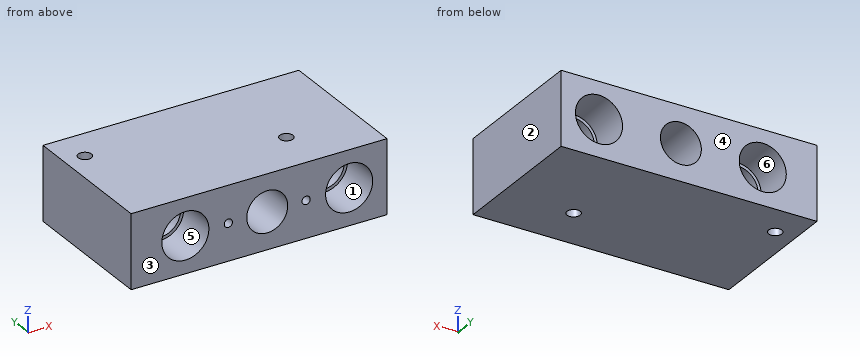
from build123d import *

# Parameters (mm, degrees)
F0_W      = 125
F0_H      = 70
F1_DEPTH  = 36
F2_R      = 10
F3_DEPTH  = 70.001
F4_R      = 11.5
F5_DEPTH  = 20
F6_R      = 11.5
F7_DEPTH  = 20
F8_R      = 3.25
F8_R_2    = 12.900097
F9_DEPTH  = 36.001
F10_R     = 2
F11_DEPTH = 20


with BuildPart() as f1:
    # F0 (on Top) → F1 (new body)
    with BuildSketch(Plane.XY):
        with Locations((62.5, 35)):
            Rectangle(F0_W, F0_H)
    extrude(amount=F1_DEPTH)

    # F2 (on face) → F3 (cut, through all)
    with BuildSketch(Plane.XZ):
        with Locations((26.5, 18)):
            Circle(F2_R)
        with Locations((66.5, 18)):
            Circle(F2_R)
        with Locations((106.5, 18)):
            Circle(F2_R)
    extrude(amount=-F3_DEPTH, mode=Mode.SUBTRACT)

    # F4 (on face) → F5 (cut)
    with BuildSketch(Plane.XZ):
        with Locations((26.5, 18)):
            Circle(F4_R)
        with Locations((106.5, 18)):
            Circle(F4_R)
    extrude(amount=-F5_DEPTH, mode=Mode.SUBTRACT)

    # F6 (on face) → F7 (cut)
    with BuildSketch(Plane(origin=(0, 70, 0), x_dir=(-1, 0, 0), z_dir=(0, 1, 0))):
        with Locations((-106.5, 18)):
            Circle(F6_R)
        with Locations((-26.5, 18)):
            Circle(F6_R)
    extrude(amount=-F7_DEPTH, mode=Mode.SUBTRACT)

    # F8 (on face) → F9 (cut, through all)
    with BuildSketch(Plane(origin=(0, 0, 0), x_dir=(1, 0, 0), z_dir=(0, 0, -1))):
        with Locations((90, -23)):
            Circle(F8_R)
        with Locations((125.049993, 12.9)):
            Circle(F8_R_2)
        with Locations((10, -53)):
            Circle(F8_R)
    extrude(amount=-F9_DEPTH, mode=Mode.SUBTRACT)

    # F10 (on face) → F11 (cut)
    with BuildSketch(Plane.XZ):
        with Locations((47.5, 18)):
            Circle(F10_R)
        with Locations((85.5, 18)):
            Circle(F10_R)
    extrude(amount=-F11_DEPTH, mode=Mode.SUBTRACT)


solid = f1.part
Work out the finished part from the listing and answer in its coordinate system (mm). Face numbers are marked on the shaded views. A direction names the side the tool comes from. Coordinates: 2 decimals unless noted, no trailing zeros. Write each loop counter-clockwise with the first axis right and the second up, starting at its lowest first coordinate (ties: lowest second). Pieces come first, ordered by that corner, then holes. Notation, with made-up numbers: M 13.5,8 L 71.5,8 A21 cw 71.5,37 Z; hole C 14,-28 d5. An arc over 180 degrees is marked long. Write item = value, one per line.
1. The part is cut by section A-A (x = 90). Determine the outline of the cut face in (y, z), then the cut area to 3 significant figures.
Solution:
outline = M 0,0 L 19.75,0 L 19.75,36 L 0,36 Z; M 26.25,0 L 70,0 L 70,36 L 26.25,36 Z
area = 2,290 mm2
2. The part is cut by section D-D (y = 35.5). Determine the outline of the cut face in (x, z).
Solution:
outline = M 0,0 L 125,0 L 125,36 L 0,36 Z; hole C 26.5,18 d20; hole C 66.5,18 d20; hole C 106.5,18 d20
3. Flat-ended cylindrical pins translate along their axes: pin 1 (3.5 mm diameter, centred on x = 47.5, z = 18, fed in from -Y); pin 2 (14 mm diameter, centred on x = 106.5, z = 18, fed in from +Y). Find the tip coordinate at first contact, or state that the pin passes through.
Solution:
pin_1 = 20
pin_2 = through
4. For the marked faces 4, 5 and 6, determine the directions among +Z, -Z, +X, -X, +Y, -Y from which every point of the face is accessible in a straight line to the end or side of a thin tool.
Solution:
face_4 = +Z, -Z, +X, -X, +Y
face_5 = -Y
face_6 = +Y
5. Straight lines are drawn through the part: line 1 (Y direction, x = 10, z = 8); line 2 (Z direction, x = 85.5, y = 12.5); line 3 (X direction, y = 19.5, z = 19.5). For each, find the intervals that lie inside material, in ascending order. Write a range as from..to.
Solution:
line_1 = 0..49.75, 56.25..70
line_2 = 0..16, 20..36
line_3 = 0..15.1, 37.9..46.18, 48.82..56.61, 76.39..84.18, 86.82..95.1, 117.9..125
6. The part is cut by section B-B (y = 53). Determine the outline of the cut face in (x, z).
Solution:
outline = M 0,0 L 6.75,0 L 6.75,36 L 0,36 Z; M 13.25,0 L 125,0 L 125,36 L 13.25,36 Z; hole C 26.5,18 d23; hole C 66.5,18 d20; hole C 106.5,18 d23
7. The part is cut by section C-C (z = 23.5). State how many separate pieces and enclosed holes the cut face has, then the cut area to 3 significant figures.
Solution:
separate_pieces = 4
enclosed_holes = 2
area = 4,900 mm2
8. Determine the mould class of the marked faces 1, 2 and 3 for opening direction X: released by +X, released by -X, zero draft, split by the parting line, or undercut.
Solution:
face_1 = undercut
face_2 = released by +X
face_3 = zero draft
